Drawing for the job (mm, zero at the part's lowest x, y, z). A direction names the side the tool comes from. Round coordinates to 2 decimals unless told otherwise and drop trailing zeros. Loops run counter-clockwise (first coordinate to the right, second up) from the corner with the lowest first, then second, coordinate; pieces in that order, holes last. Notation, with made-up numbers: M 15.5,42 L 45.5,42 A27 cw 45.5,72 Z; hole C 64,5 d9. An arc over 180 degrees is marked long. Answer in a Markdown table with one row per item.
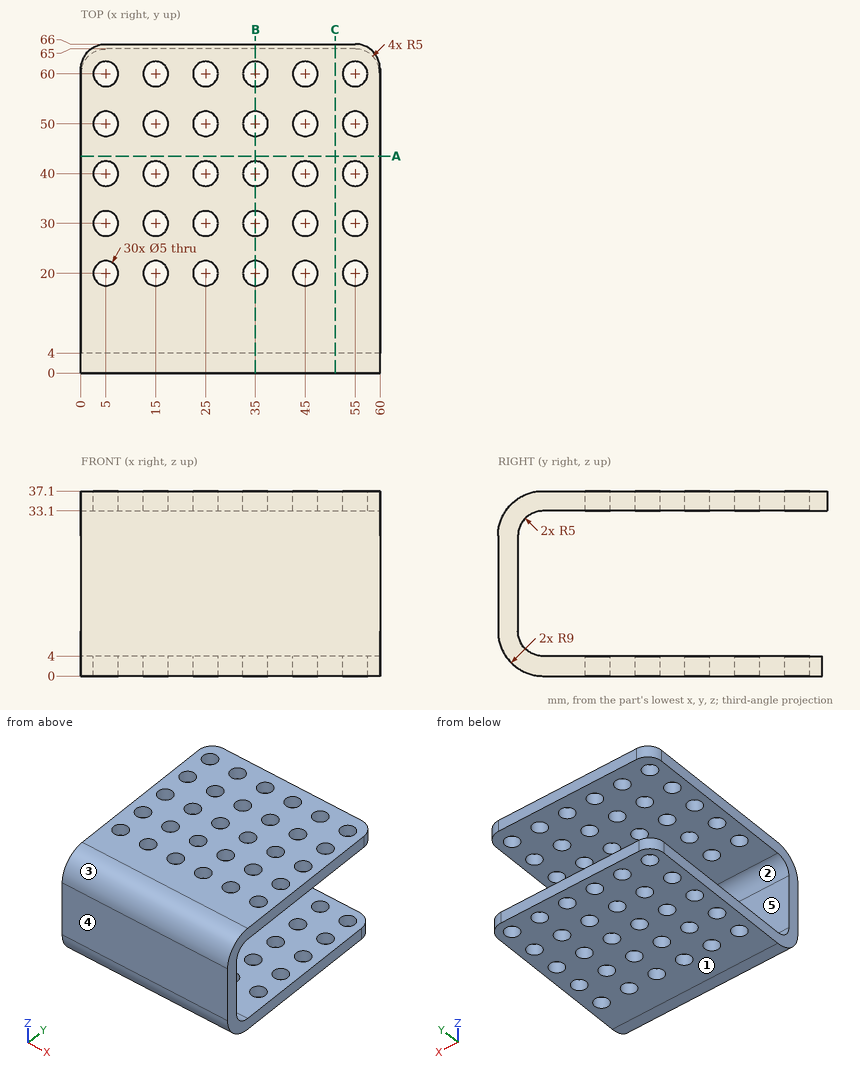
1. Mould opens along Z. For the marked faces 1, 2 and 3 say: +Z half, -Z half, draft (parallel to the pull), parting line (faces both ways), or undercut.
Verdict:
| item | result |
|---|---|
| face 1 | -Z half |
| face 2 | undercut |
| face 3 | +Z half |
2. Tool access for the marked faces 4 and 5: list every direction of +Z, -Z, +X, -X, +Y, -Y with a clear straight run to the whole face (end or side of a thin tool).
Verdict:
| item | result |
|---|---|
| face 4 | +Z, -Z, +X, -X, -Y |
| face 5 | +X, -X, +Y |
3. Saw through at A-A (y = 43.5). Write the cut outline in (x, z), and give its area (3 significant figures).
Verdict:
| item | result |
|---|---|
| outline | M 0,0 L 60,0 L 60,4 L 0,4 Z; M 0,33.1 L 60,33.1 L 60,37.1 L 0,37.1 Z |
| area | 480 mm² |
4. Saw through at B-B (x = 35). State how many separate pieces and enclosed holes the cut face has, and give its area (3 significant figures).
Verdict:
| item | result |
|---|---|
| separate pieces | 11 |
| enclosed holes | 0 |
| area | 416 mm² |
5. Saw through at C-C (x = 51). Write the cut outline in (y, z), and give its area (3 significant figures).
Verdict:
| item | result |
|---|---|
| outline | M 0,9 A9 ccw 9,0 L 65,0 L 65,4 L 9,4 A5 cw 4,9 L 4,28.1 A5 cw 9,33.1 L 66,33.1 L 66,37.1 L 9,37.1 A9 ccw 0,28.1 Z |
| area | 616 mm² |
6. Wall check: probe 1 along Z at (x, y) = (29.5, 34.5); probe 2 along Y at (x, z) = (33.5, 35.5); probe 3 along Y at (x, z) = (57, 3.5). Give the ranges that are in metal, low to high.
Verdict:
| item | result |
|---|---|
| probe 1 | z = 0 to 4, 33.1 to 37.1 |
| probe 2 | y = 3.88 to 18, 22 to 28, 32 to 38, 42 to 48, 52 to 58, 62 to 66 |
| probe 3 | y = 1.88 to 18.5, 21.5 to 28.5, 31.5 to 38.5, 41.5 to 48.5, 51.5 to 58.5, 61.5 to 64.58 |
7. Pin check, flat tips, straight feed: pin 1 (9.5 mm diameter, centred on x = 37, z = 22, fed in from +Y); pin 2 (3 mm diameter, centred on x = 35, y = 50, fed in from +Z). Stop position of each tip, or through.
Verdict:
| item | result |
|---|---|
| pin 1 | stops at y = 4 |
| pin 2 | passes through |
